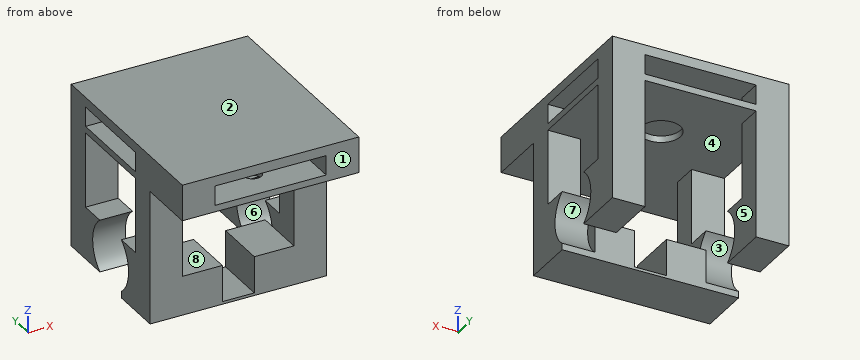
```python
from build123d import *

# Parameters (mm, degrees)
SKETCH1_W           = 68.58
SKETCH1_H           = 55.88
BOSS_EXTRUDE1_DEPTH = 3.81
SKETCH2_W           = 12.7
SKETCH2_H           = 10.16
BOSS_EXTRUDE2_DEPTH = 59.69
SKETCH6_W           = 12.7
SKETCH6_H           = 20.32
BOSS_EXTRUDE3_DEPTH = 35.56
SKETCH4_R           = 12.7
CUT_EXTRUDE1_DEPTH  = 107.717790925
SKETCH7_W           = 68.58
SKETCH7_H           = 55.88
SKETCH7_W_2         = 43.18
SKETCH7_H_2         = 22.86
BOSS_EXTRUDE4_DEPTH = 2.54
SKETCH8_R           = 3.429
SKETCH8_R_2         = 7.493
CUT_EXTRUDE2_DEPTH  = 2.54
SKETCH9_W           = 68.58
SKETCH9_H           = 20.32
BOSS_EXTRUDE5_DEPTH = 2.54
CUT_EXTRUDE3_REACH  = 110.159
SKETCH10_W          = 12.446
SKETCH10_H          = 3.048
SKETCH11_W          = 15.367
SKETCH11_H          = 20.32
BOSS_EXTRUDE6_DEPTH = 12.7
BOSS_EXTRUDE7_DEPTH = 22.86


with BuildPart() as part:
    # Sketch1 → Boss-Extrude1 (new body)
    with BuildSketch(Plane.XY):
        with Locations((34.29, 27.94)):
            Rectangle(SKETCH1_W, SKETCH1_H)
    extrude(amount=BOSS_EXTRUDE1_DEPTH)

    # Sketch2 → Boss-Extrude2 (add)
    with BuildSketch(Plane(origin=(0, 0, 0), x_dir=(-1, 0, 0), z_dir=(0, 0, -1))):
        with Locations((-62.23, 50.8)):
            Rectangle(SKETCH2_W, SKETCH2_H)
        with Locations((-6.35, 50.8)):
            Rectangle(SKETCH2_W, SKETCH2_H)
        with Locations((-6.35, 5.08)):
            Rectangle(SKETCH2_W, SKETCH2_H)
        with Locations((-62.23, 5.08)):
            Rectangle(SKETCH2_W, SKETCH2_H)
    extrude(amount=BOSS_EXTRUDE2_DEPTH)

    # Sketch6 → Boss-Extrude3 (add)
    with BuildSketch(Plane(origin=(0, 10.16, 0), x_dir=(1, 0, 0), z_dir=(0, 1, 0))):
        with Locations((62.23, 49.53)):
            Rectangle(SKETCH6_W, SKETCH6_H)
        with Locations((6.35, 49.53)):
            Rectangle(SKETCH6_W, SKETCH6_H)
    extrude(amount=BOSS_EXTRUDE3_DEPTH)

    # Sketch4 → Cut-Extrude1 (cut, through all)
    with BuildSketch(Plane(origin=(68.58, 0, 0), x_dir=(0, 0, -1), z_dir=(1, 0, 0))):
        with Locations((49.53, 27.94)):
            Circle(SKETCH4_R)
    extrude(amount=-CUT_EXTRUDE1_DEPTH, mode=Mode.SUBTRACT)

    # Sketch7 → Boss-Extrude4 (add)
    with BuildSketch(Plane(origin=(0, 0, -7.62), x_dir=(-1, 0, 0), z_dir=(0, 0, -1))):
        with Locations((-34.29, 27.94)):
            Rectangle(SKETCH7_W, SKETCH7_H)
        with Locations((-34.29, -11.43)):
            Rectangle(SKETCH7_W_2, SKETCH7_H_2)
    extrude(amount=BOSS_EXTRUDE4_DEPTH)

    # Sketch8 → Cut-Extrude2 (cut)
    with BuildSketch(Plane(origin=(0, 0, -10.16), x_dir=(-1, 0, 0), z_dir=(0, 0, -1))):
        with Locations((-34.29, -10.16)):
            Circle(SKETCH8_R)
        with Locations((-34.29, 27.94)):
            Circle(SKETCH8_R_2)
    extrude(amount=-CUT_EXTRUDE2_DEPTH, mode=Mode.SUBTRACT)

    # Sketch9 → Boss-Extrude5 (add)
    with BuildSketch(Plane(origin=(0, 0, -59.69), x_dir=(-1, 0, 0), z_dir=(0, 0, -1))):
        with Locations((-34.29, 10.16)):
            Rectangle(SKETCH9_W, SKETCH9_H)
    extrude(amount=BOSS_EXTRUDE5_DEPTH)

    # Sketch10 → Cut-Extrude3 (cut, up to next)
    with BuildSketch(Plane.XZ, mode=Mode.PRIVATE) as cut_extrude3_sk1:
        with Locations((34.29, -59.69)):
            Rectangle(SKETCH10_W, SKETCH10_H)
    cut_extrude3_tool1 = extrude(cut_extrude3_sk1.sketch, amount=-CUT_EXTRUDE3_REACH, mode=Mode.PRIVATE) & part.part
    add(cut_extrude3_tool1.solids().sort_by_distance((34.29, 0, -59.69))[0], mode=Mode.SUBTRACT)

    # Sketch11 → Boss-Extrude6 (add)
    with BuildSketch(Plane.XY.offset(-59.69)):
        with Locations((20.3835, 10.16)):
            Rectangle(SKETCH11_W, SKETCH11_H)
        with Locations((48.1965, 10.16)):
            Rectangle(SKETCH11_W, SKETCH11_H)
    extrude(amount=BOSS_EXTRUDE6_DEPTH)

    # Sketch12 → Boss-Extrude7 (add)
    with BuildSketch(Plane.XZ):
        Polygon((12.7, -10.16), (0, -10.16), (0, 3.81), (68.58, 3.81), (68.58, -10.16), (55.88, -10.16), (55.88, 0), (12.7, 0), align=None)
    extrude(amount=BOSS_EXTRUDE7_DEPTH)


solid = part.part
```
Work out the finished part from the listing and answer in its coordinate system (mm). Face numbers are marked on the shaded views. A direction names the side the tool comes from. Round coordinates to 2 decimals unless told otherwise and drop trailing zeros. Order: outer loops, then holes, each group sorted by start corner. A loop starts at its lowest first (then second) coordinate and runs counter-clockwise, first axis right, second up.
Q1. A cutting plane is placed at D-D, the plane x = 4.5. Determine the outline of the cut face in (y, z).
Solution:
outline: (-22.86, -10.16) - (0, -10.16) - (0, -62.23) - (20.32, -62.23) - (20.32, -59.69) arc R12.7 cw to (20.32, -39.37) - (10.16, -39.37) - (10.16, -10.16) - (45.72, -10.16) - (45.72, -39.37) - (35.56, -39.37) arc R12.7 cw to (35.56, -59.69) - (55.88, -59.69) - (55.88, 3.81) - (-22.86, 3.81) - close; hole (10.16, -7.62) - (45.72, -7.62) - (45.72, 0) - (10.16, 0) - close
Q2. Find the intervals of material crossed by line 1 along Y through (x, z) = (34.29, -9.25); line 2 along Z through (x, y) = (39, 10); line 3 along Z through (x, y) = (58.5, 29.5), in increasing order.
Solution:
line 1: y = -22.86 to -13.59, -6.73 to 20.45, 35.43 to 55.88
line 2: z = -62.23 to -61.21, -10.16 to -7.62, 0 to 3.81
line 3: z = -10.16 to -7.62, 0 to 3.81
Q3. A cutting plane is placed at A-A, the plane x = 23. Determine the outline of the cut face in (y, z), then the cut area to 3 significant figures.
Solution:
outline: (-22.86, -10.16) - (55.88, -10.16) - (55.88, -7.62) - (-22.86, -7.62) - close; (-22.86, 0) - (55.88, 0) - (55.88, 3.81) - (-22.86, 3.81) - close; (0, -62.23) - (20.32, -62.23) - (20.32, -46.99) - (0, -46.99) - close
area: 810 mm2
Q4. A cutting plane is placed at C-C, the plane z = -13.5. Determine the outline of the cut face in (x, y), then the cut area to 3 significant figures.
Solution:
outline: (0, 0) - (12.7, 0) - (12.7, 10.16) - (0, 10.16) - close; (0, 45.72) - (12.7, 45.72) - (12.7, 55.88) - (0, 55.88) - close; (55.88, 0) - (68.58, 0) - (68.58, 10.16) - (55.88, 10.16) - close; (55.88, 45.72) - (68.58, 45.72) - (68.58, 55.88) - (55.88, 55.88) - close
area: 516 mm2
Q5. A tool of negligible diameter and unlimited length cuts with its end or side. For the marked faces 4, 5, 6, 7 and 8, from which of +Z, -Z, +X, -X, +Y, -Y can it reach the whole face along a straight path? Write none if from no direction.
Solution:
face 4: none
face 5: -Z, +Y
face 6: +X, -X
face 7: +X
face 8: +Y, -Y
Q6. A cutting plane is placed at B-B, the plane y = -5.5. Determine the outline of the cut face in (x, z), then the cut area to 3 significant figures.
Solution:
outline: (0, -10.16) - (68.58, -10.16) - (68.58, 3.81) - (0, 3.81) - close; hole (12.7, -7.62) - (55.88, -7.62) - (55.88, 0) - (12.7, 0) - close
area: 629 mm2
Q7. Given pin 1 Ø12 at (x, y) = (34.29, 27.94) entering from -Z; pin 2 Ø10 at (y, z) = (10.5, -35) entering from -X; pin 3 Ø1.5 at (x, y) = (41, 45) entering from -Z; pin 4 Ø2 at (x, z) = (47, -47.5) entering from -Y, each flat-ended and moving along its own axis, determine where each tip first touches the part or whether it passes through.
Solution:
pin 1: stops at z = 0
pin 2: stops at x = 0
pin 3: stops at z = -10.16
pin 4: stops at y = 0
Q8. The mould has two halves that part along Y. Classify the marked faces 1, 2 and 3: pulls with the +Y half, pulls with the -Y half, needs draft (parallel to the pull), parting line crosses it, or undercut.
Solution:
face 1: pulls with the -Y half
face 2: needs draft
face 3: undercut
